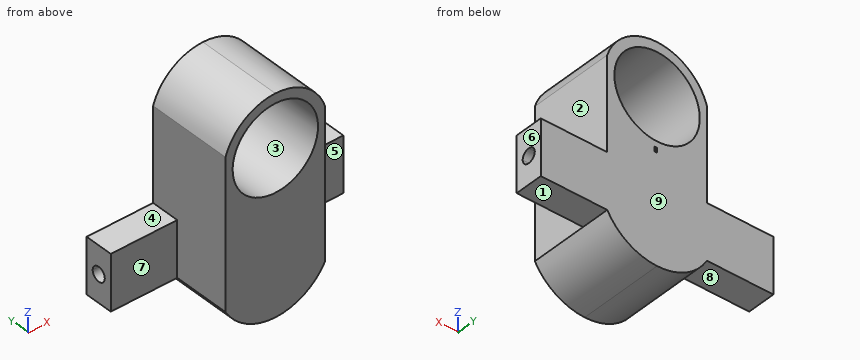
from build123d import *

# Parameters (mm, degrees)
SKETCH1_W           = 21
SKETCH1_H           = 45.065175024
BOSS_EXTRUDE1_DEPTH = 18
SKETCH6_R           = 9
CUT_EXTRUDE4_DEPTH  = 52
CUT_EXTRUDE5_DEPTH  = 52
SKETCH10_W          = 5.809475019
SKETCH10_H          = 6
BOSS_EXTRUDE2_DEPTH = 14
SKETCH11_W          = 0.5
SKETCH11_H          = 1
CUT_EXTRUDE6_DEPTH  = 0.5
CUT_EXTRUDE7_DEPTH  = 10


with BuildPart() as part:
    # Sketch1 → Boss-Extrude1 (new body)
    with BuildSketch(Plane(origin=(0, 0, 0), x_dir=(1, 0, 0), z_dir=(0, 1, 0))):
        with Locations((0, -10.532587512)):
            Rectangle(SKETCH1_W, SKETCH1_H)
    extrude(amount=BOSS_EXTRUDE1_DEPTH)

    # Sketch6 → Cut-Extrude4 (cut)
    with BuildSketch(Plane(origin=(0, 18, 0), x_dir=(1, 0, 0), z_dir=(0, 1, 0))):
        with BuildLine():
            Line((0, -33.065175024), (10.5, -33.065175024))
            Line((10.5, -33.065175024), (10.5, -25.343894287))
            ThreePointArc((10.5, -25.343894287), (6.51667431, -30.927057214), (0, -33.065175024))
        make_face()
        with Locations(Location((0, -22.065175024, 0), (0, 0, 270))):
            Circle(SKETCH6_R)
        with BuildLine():
            Line((-10.5, -33.065175024), (0, -33.065175024))
            ThreePointArc((0, -33.065175024), (-6.51667431, -30.927057214), (-10.5, -25.343894287))
            Line((-10.5, -25.343894287), (-10.5, -33.065175024))
        make_face()
    extrude(amount=-CUT_EXTRUDE4_DEPTH, mode=Mode.SUBTRACT)

    # Sketch8 → Cut-Extrude5 (cut)
    with BuildSketch(Plane(origin=(0, 18, 0), x_dir=(1, 0, 0), z_dir=(0, 1, 0))):
        with BuildLine():
            Line((0, 12), (-10.5, 12))
            Line((-10.5, 12), (-10.5, 5.809475019))
            ThreePointArc((-10.5, 5.809475019), (-6.094518019, 10.337158706), (0, 12))
        make_face()
        with BuildLine():
            Line((10.5, 12), (0, 12))
            ThreePointArc((0, 12), (6.094518019, 10.337158706), (10.5, 5.809475019))
            Line((10.5, 5.809475019), (10.5, 12))
        make_face()
    extrude(amount=-CUT_EXTRUDE5_DEPTH, mode=Mode.SUBTRACT)

    # Sketch10 → Boss-Extrude2 (add)
    with BuildSketch(Plane.ZY.offset(10.5)):
        with Locations((2.90473751, 15)):
            Rectangle(SKETCH10_W, SKETCH10_H)
        with Locations((-2.90473751, 15)):
            Rectangle(SKETCH10_W, SKETCH10_H)
    boss_extrude2 = extrude(amount=BOSS_EXTRUDE2_DEPTH)

    # Sketch11 → Cut-Extrude6 (cut)
    with BuildSketch(Plane(origin=(0, 18, 0), x_dir=(1, 0, 0), z_dir=(0, 1, 0))):
        with Locations((0.25, -11.282587512)):
            Rectangle(SKETCH11_W, SKETCH11_H)
    extrude(amount=-CUT_EXTRUDE6_DEPTH, mode=Mode.SUBTRACT)

    # Mirror1: Boss-Extrude2 across plane
    add(boss_extrude2.mirror(Plane(origin=(0, 17.5, 0), x_dir=(0, 0, 1), z_dir=(-1, 0, 0))))

    # Sketch12 → Cut-Extrude7 (cut)
    with BuildSketch(Plane.ZY.offset(24.5)):
        with BuildLine():
            ThreePointArc((1.5, 15), (1.060660172, 16.060660172), (0, 16.5))
            Line((0, 16.5), (0, 13.5))
            ThreePointArc((0, 13.5), (1.060660172, 13.939339828), (1.5, 15))
        make_face()
        with BuildLine():
            Line((0, 13.5), (0, 16.5))
            ThreePointArc((0, 16.5), (-1.5, 15), (0, 13.5))
        make_face()
    cut_extrude7 = extrude(amount=-CUT_EXTRUDE7_DEPTH, mode=Mode.SUBTRACT)

    # Mirror2: Cut-Extrude7 across plane
    add(cut_extrude7.mirror(Plane(origin=(0, 17.5, 0), x_dir=(0, 0, 1), z_dir=(-1, 0, 0))), mode=Mode.SUBTRACT)


solid = part.part
Work out the finished part from the listing and answer in its coordinate system (mm). Face numbers are marked on the shaded views. A direction names the side the tool comes from. Give positions to 0.01 mm unless a question says otherwise; leave off trailing zeros. Order: outer loops, then holes, each group sorted by start corner. A loop starts at its lowest first (then second) coordinate and runs counter-clockwise, first axis right, second up. Notation, with made-up numbers: (11.5, 71.5) -> (19.5, 71.5) arc R28 ccw to (19.5, 103.5) -> close; hole circle Ø5 at (-14.5, -21.75). An arc over 180 degrees is marked (long way). Answer as a JSON object with one key per item and string values. Group by question number.
1. Section B-B on z = 29 is taken. Determine the outline of the cut face in (x, y).
2. Flat-ended cylindrical pins translate along their axes: pin 1 Ø6 at (x, z) = (-18, 1) entering from -Y; pin 2 Ø5 at (x, y) = (-16, 15.5) entering from -Z; pin 3 Ø6 at (x, y) = (16.5, 12) entering from +Z. Find the tip coordinate at first contact, or state that the pin passes through.
3. Section C-C on x = 15.5 is taken. Determine the outline of the cut face in (y, z).
4. Section A-A on y = 5.5 is taken. Determine the outline of the cut face in (x, z).
5. The mould has two halves that part along Z. Classify the marked faces 1, 2, 3 and 4: released by +Z, released by -Z, zero draft, split by the parting line, or undercut.
6. Section D-D on x = -2 is taken. Determine the outline of the cut face in (y, z).
7. A tool of negligible diameter and unlimited length cuts with its end or side. For the marked faces 5, 6, 7, 8 and 9, from which of +Z, -Z, +X, -X, +Y, -Y can it reach the whole face along a straight path? Write none if from no direction.
8. Consider line 1 along Y through (x, z) = (18, 4.5); line 2 along X through (y, z) = (1.25, -5.5); line 3 along X through (y, z) = (8, 26.5). Determine where each line is inside the solid, lowest interval first. Write a range as [from, to].
Result sheet:
{
 "1": {"outline": "(-8.54, 0) -> (-5.74, 0) -> (-5.74, 18) -> (-8.54, 18) -> close; (5.74, 0) -> (8.54, 0) -> (8.54, 18) -> (5.74, 18) -> close"},
 "2": {"pin 1": "stops at y = 12", "pin 2": "stops at z = -5.81", "pin 3": "stops at z = 5.81"},
 "3": {"outline": "(12, -5.81) -> (18, -5.81) -> (18, 5.81) -> (12, 5.81) -> close; hole circle Ø3 at (15, 0)"},
 "4": {"outline": "(-10.5, -5.81) arc R12 ccw to (10.5, -5.81) -> (10.5, 25.34) arc R11 ccw to (-10.5, 25.34) -> close; hole circle Ø18 at (0, 22.07)"},
 "5": {"face 1": "released by -Z", "face 2": "zero draft", "face 3": "undercut", "face 4": "released by +Z"},
 "6": {"outline": "(0, -11.83) -> (18, -11.83) -> (18, 13.29) -> (0, 13.29) -> close; (0, 30.84) -> (18, 30.84) -> (18, 32.88) -> (0, 32.88) -> close"},
 "7": {"face 5": "+Z, -Z, +X, -Y", "face 6": "+Z, -Z, +X, +Y, -Y", "face 7": "+Z, -Z, -X, -Y", "face 8": "-Z, -X, +Y, -Y", "face 9": "+Z, -Z, +X, -X, +Y"},
 "8": {"line 1": "y = [12, 18]", "line 2": "x = [-10.5, 10.5]", "line 3": "x = [-10.07, -7.83], [7.83, 10.07]"}
}
